Verification items for the finished model (mm, model axes). Face numbers are marked on the shaded views. Round coordinates to 2 decimals unless told otherwise and drop trailing zeros. Order: outer loops, then holes, each group sorted by start corner. A loop starts at its lowest first (then second) coordinate and runs counter-clockwise, first axis right, second up. Notation, with made-up numbers: (-6, 45) -> (41, 45) arc R21 ccw to (41, 75) -> close; hole circle Ø10 at (53.5, 18.25). An arc over 180 degrees is marked (long way). Write item = value, one per line. Start each with the question number.
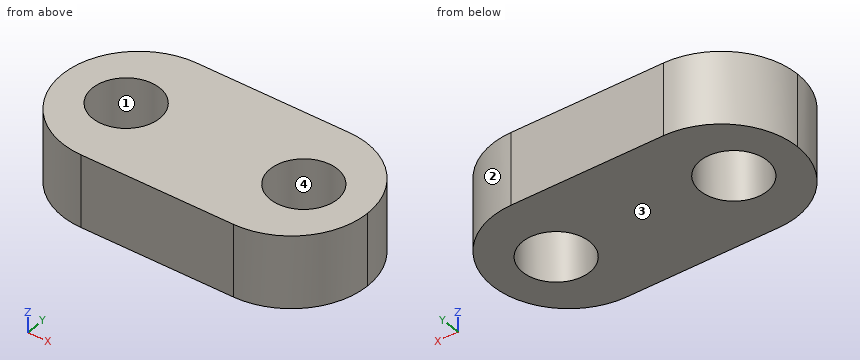
from build123d import *

# Parameters (mm, degrees)
F0_W     = 20
F0_H     = 10
F1_DEPTH = 4.75
F2_D     = 4.4
F2_DEPTH = 25
F2_TIP   = 1.3218933619
F3_R     = 4.99999


# Not quite as in the source:
# - a fillet or chamfer is up to 0.001 mm smaller than in the source, because OpenCascade refuses the exact size


with BuildPart() as f1:
    # F0 (on Top) → F1 (new body)
    with BuildSketch(Plane.XY):
        Rectangle(F0_W, F0_H)
    extrude(amount=F1_DEPTH)

    # F2
    with Locations(Plane(origin=(0, 0, 0), x_dir=(1, 0, 0), z_dir=(0, 0, -1))):
        with Locations((-5.82, 0), (5.82, 0)):
            Hole(F2_D / 2, depth=F2_DEPTH)
            with Locations((0, 0, -(F2_DEPTH + F2_TIP / 2))):  # 118° drill point
                Cone(0, F2_D / 2, F2_TIP, mode=Mode.SUBTRACT)

    # F3 (radius 5 in the source; OpenCascade refuses exactly that, so slightly less here)
    f3_edges = [f1.edges().sort_by_distance(p)[0] for p in [
        (10, 5, 2.375),
        (10, -5, 2.375),
        (-10, 5, 2.375),
        (-10, -5, 2.375),
    ]]
    fillet(f3_edges, radius=F3_R)


solid = f1.part
(1) Scan lines: line 1 along X through (y, z) = (0.75, 2.25); line 2 along Y through (x, z) = (6.75, 3.6); line 3 along Y through (x, z) = (-5.75, 4.45). Record each from-to range of solid material in increasing order. Write a range as from..to.
(2) Cross-section at B-B (x = -4). Enter the section's corners in (y, z), and give its area (3 significant figures).
(3) Cross-section at D-D (x = -7.25). Enter the section's corners in (y, z).
(4) Cross-section at C-C (y = -1.75). Enter the section's corners in (x, z).
(5) Draft check along X on the marked faces 1, 2, 3 and 4. Enter one of: +X half, -X half, draft (parallel to the pull), parting line (faces both ways), or undercut.
(6) Cross-section at A-A (z = 2.3). Give the number of separate pieces and of enclosed holes in the cut face, and give its area (3 significant figures).
(7) Depth check by flat-ended pin: pin 1 (1 mm diameter, centred on x = 7, y = 1, fed in from -Z). Enter the tip coordinate at first touch or a pass-through.
Outcome:
q1.line_1 = -9.94..-7.89, -3.75..3.75, 7.89..9.94
q1.line_2 = -4.68..-1.99, 1.99..4.68
q1.line_3 = -4.94..-2.2, 2.2..4.94
q2.outline = (-5, 0) -> (-1.24, 0) -> (-1.24, 4.75) -> (-5, 4.75) -> close; (1.24, 0) -> (5, 0) -> (5, 4.75) -> (1.24, 4.75) -> close
q2.area = 35.8 mm^2
q3.outline = (-4.47, 0) -> (-1.67, 0) -> (-1.67, 4.75) -> (-4.47, 4.75) -> close; (1.67, 0) -> (4.47, 0) -> (4.47, 4.75) -> (1.67, 4.75) -> close
q4.outline = (-9.68, 0) -> (-7.15, 0) -> (-7.15, 4.75) -> (-9.68, 4.75) -> close; (-4.49, 0) -> (4.49, 0) -> (4.49, 4.75) -> (-4.49, 4.75) -> close; (7.15, 0) -> (9.68, 0) -> (9.68, 4.75) -> (7.15, 4.75) -> close
q5.face_1 = undercut
q5.face_2 = +X half
q5.face_3 = draft
q5.face_4 = undercut
q6.separate_pieces = 1
q6.enclosed_holes = 2
q6.area = 148 mm^2
q7.pin_1 = through
